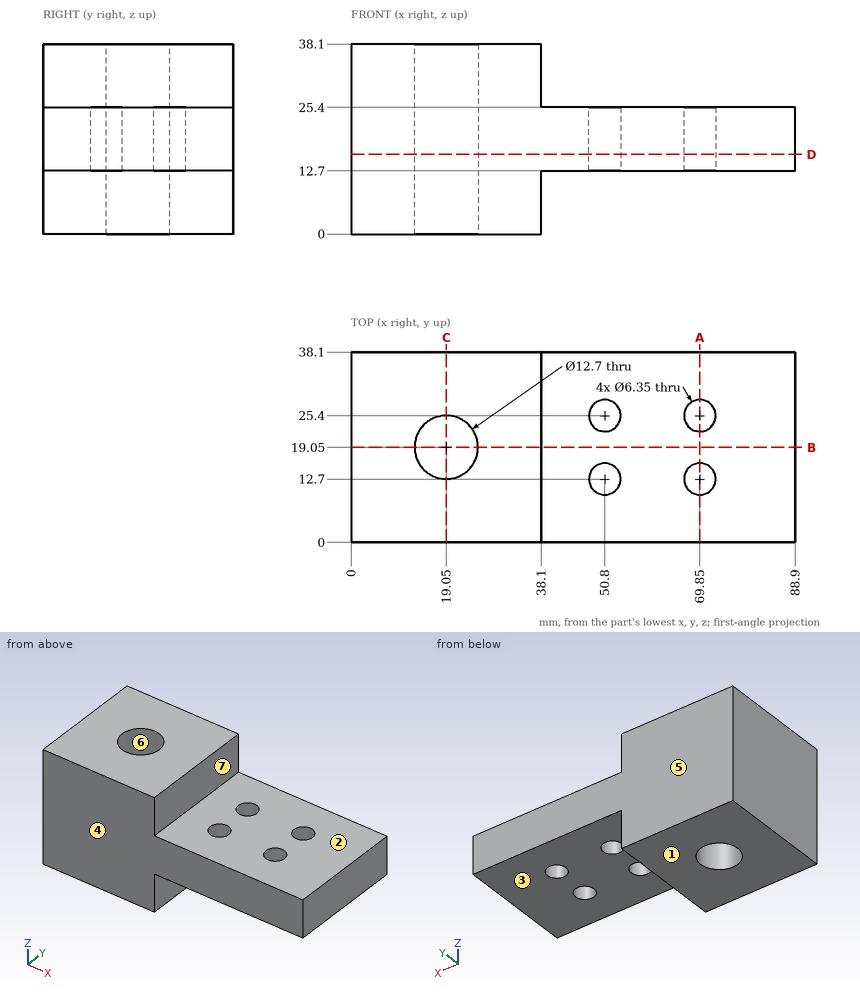
The figure shows three views and two pictorial views of one solid part (mm, origin at its lowest corner). Answer the questions. A direction names the side the tool comes from. Give positions to 0.01 mm unless a question says otherwise; leave off trailing zeros. Loops run counter-clockwise (first coordinate to the right, second up) from the corner with the lowest first, then second, coordinate; pieces in that order, holes last. Notation, with made-up numbers: M 38,80.25 L 81,80.25 A11 ccw 81,85.25 Z; hole C -19,77 d9. An arc over 180 degrees is marked long. Write each question's results on one line, items separated by ' | '.
1. Given pin 1 (8.5 mm diameter, centred on x = 50.8, y = 25.4, fed in from -Z); pin 2 (6.5 mm diameter, centred on y = 20, z = 29.5, fed in from +X); pin 3 (3 mm diameter, centred on x = 72.5, y = 12, fed in from +Z), each flat-ended and moving along its own axis, determine where each tip first touches the part or whether it passes through.
Values:
pin 1: stops at z = 12.7 | pin 2: stops at x = 38.1 | pin 3: stops at z = 25.4
2. The mould has two halves that part along Y. Classify the marked faces 4, 5, 6 and 7: pulls with the +Y half, pulls with the -Y half, needs draft (parallel to the pull), parting line crosses it, or undercut.
Values:
face 4: pulls with the -Y half | face 5: pulls with the +Y half | face 6: undercut | face 7: needs draft
3. Section B-B on y = 19.05 is taken. Give the vertices of the cut face in (x, z).
Values:
outline: M 0,0 L 12.7,0 L 12.7,38.1 L 0,38.1 Z; M 25.4,0 L 38.1,0 L 38.1,12.7 L 88.9,12.7 L 88.9,25.4 L 38.1,25.4 L 38.1,38.1 L 25.4,38.1 Z
4. Section A-A on x = 69.85 is taken. Give the vertices of the cut face in (y, z) (3 decimals).
Values:
outline: M 0,12.7 L 9.525,12.7 L 9.525,25.4 L 0,25.4 Z; M 15.875,12.7 L 22.225,12.7 L 22.225,25.4 L 15.875,25.4 Z; M 28.575,12.7 L 38.1,12.7 L 38.1,25.4 L 28.575,25.4 Z
5. Straight lines are drawn through the part: line 1 (Y direction, x = 50.8, z = 18) (3 decimals); line 2 (Y direction, x = 50, z = 22); line 3 (X direction, y = 10, z = 16.5). For each, find the intervals that lie inside material, in ascending order. Write a range as [from, to].
Values:
line 1: y = [0, 9.525], [15.875, 22.225], [28.575, 38.1] | line 2: y = [0, 9.63], [15.77, 22.33], [28.47, 38.1] | line 3: x = [0, 49.13], [52.47, 68.18], [71.52, 88.9]
6. Section C-C on x = 19.05 is taken. Give the vertices of the cut face in (y, z), plus the area to 3 significant figures.
Values:
outline: M 0,0 L 12.7,0 L 12.7,38.1 L 0,38.1 Z; M 25.4,0 L 38.1,0 L 38.1,38.1 L 25.4,38.1 Z | area: 968 mm^2
7. A tool of negligible diameter and unlimited length cuts with its end or side. For the marked faces 1, 2 and 3, from which of +Z, -Z, +X, -X, +Y, -Y can it reach the whole face along a straight path? Write none if from no direction.
Values:
face 1: -Z, +X, -X, +Y, -Y | face 2: +Z, +X, +Y, -Y | face 3: -Z, +X, +Y, -Y
8. Section D-D on z = 16 is taken. Give the vertices of the cut face in (x, y) (3 decimals), plus the area to 3 significant figures.
Values:
outline: M 0,0 L 88.9,0 L 88.9,38.1 L 0,38.1 Z; hole C 19.05,19.05 d12.7; hole C 50.8,12.7 d6.35; hole C 50.8,25.4 d6.35; hole C 69.85,12.7 d6.35; hole C 69.85,25.4 d6.35 | area: 3,130 mm^2
